```python
from build123d import *

# Parameters (mm, degrees)
F1_DEPTH = 60
F2_R     = 5
F3_R     = 25.0723290406
F4_DEPTH = 30


# Not quite as in the source:
# - a feature names something its author has since deleted; it is built from what else it names


with BuildPart() as f1:
    # F0 (on Front) → F1 (new body)
    with BuildSketch(Plane.XZ):
        with BuildLine():
            Line((21.3254676014, 72.3460770576), (-18.6745323986, 72.3460770576))
            ThreePointArc((-18.6745323986, 72.3460770576), (-39.8877358342, 63.5592804932), (-48.6745323986, 42.3460770576))
            Line((-48.6745323986, 42.3460770576), (-48.6745323986, 2.3460770576))
            ThreePointArc((-48.6745323986, 2.3460770576), (-39.8877358342, -18.867126378), (-18.6745323986, -27.6539229424))
            Line((-18.6745323986, -27.6539229424), (21.3254676014, -27.6539229424))
            ThreePointArc((21.3254676014, -27.6539229424), (42.538671037, -18.867126378), (51.3254676014, 2.3460770576))
            Line((51.3254676014, 2.3460770576), (51.3254676014, 42.3460770576))
            ThreePointArc((51.3254676014, 42.3460770576), (42.538671037, 63.5592804932), (21.3254676014, 72.3460770576))
        make_face()
    extrude(amount=F1_DEPTH)

    # F2
    f2_edges = [f1.edges().sort_by_distance(p)[0] for p in [
        (51.325468, -30, 42.346077),
        (21.325468, -30, 72.346077),
        (42.538671, 0, 63.55928),
        (42.538671, -60, 63.55928),
    ]]
    fillet(f2_edges, radius=F2_R)

    # F3 (on face) → F4 (cut)
    with BuildSketch(Plane.XZ.offset(60)):
        with Locations((-0.98494126, 18.3436237276)):
            Circle(F3_R)
    extrude(amount=-F4_DEPTH, mode=Mode.SUBTRACT)


solid = f1.part
```
Read the model definition and answer for the solid it produces. Units are mm, in the model's axes. A direction names the side the tool comes from. Give positions to 0.01 mm unless a question says otherwise; leave off trailing zeros. Loops run counter-clockwise (first coordinate to the right, second up) from the corner with the lowest first, then second, coordinate; pieces in that order, holes last.
Item 1: The part is cut by section C-C (y = -38.5). Write down the section's boundary in (x, z).
Item 2: Find the intervals of material crossed by line 1 along Z through (x, y) = (-9.5, -48.5); line 2 along Z through (x, y) = (-10, -43); line 3 along Y through (x, z) = (-11, 26.5), in increasing order.
Item 3: The mould has two halves that part along Z. Classify faces 3 (the cylindrical face through (22.93, -45.21, 25.87)), 4 (the cylindrical face through (49.9, -58.496, 22.626)), 5 (the cylindrical face through (1.045, -1.504, 70.92)): released by +Z, released by -Z, zero draft, split by the parting line, or undercut.
Item 4: Each of these flat-tipped pins is pushed along its axis until it touches: pin 1 Ø10 at (y, z) = (-29, -11.5) entering from +X; pin 2 Ø8 at (x, y) = (-32, -16) entering from +Z; pin 3 Ø12 at (y, z) = (-47, 54) entering from -X. Where does it stop, or does it pass through?
Item 5: The part is cut by section D-D (x = 17.5). Write down the section's boundary in (y, z).
Item 6: For faces 1 (the cylindrical face through (-47.249, -1.504, 22.066)), 2 (the flat face through (-1, -30, 19)), determine the directions among +Z, -Z, +X, -X, +Y, -Y from which every point of the face is accessible in a straight line to the end or side of a thin tool.
Item 7: The part is cut by section A-A (y = -27.5). Write down the section's boundary in (x, z).
Item 8: The part is cut by section B-B (z = 6.5). Write down the section's boundary in (x, y), and give its area (3 significant figures).
Taken from the geometry:
1. outline: (-48.67, 2.35) arc R30 ccw to (-18.67, -27.65) - (21.33, -27.65) arc R30 ccw to (51.33, 2.35) - (51.33, 42.35) arc R30 ccw to (21.33, 72.35) - (-18.67, 72.35) arc R30 ccw to (-48.67, 42.35) - close; hole circle Ø50.14 at (-0.98, 18.34)
2. line 1: z = -27.65 to -5.24, 41.93 to 72.35
2. line 2: z = -27.65 to -5.05, 41.74 to 72.35
2. line 3: y = -30 to 0
3. face 3: undercut
3. face 4: zero draft
3. face 5: released by +Z
4. pin 1: stops at x = 49.99
4. pin 2: stops at z = 70.86
4. pin 3: stops at x = -48.14
5. outline: (-60, -22.65) arc R5 ccw to (-55, -27.65) - (-5, -27.65) arc R5 ccw to (0, -22.65) - (0, 67.35) arc R5 ccw to (-5, 72.35) - (-55, 72.35) arc R5 ccw to (-60, 67.35) - (-60, 35.28) - (-30, 35.28) - (-30, 1.4) - (-60, 1.4) - close
6. face 1: +Z, -Z, -X, +Y
6. face 2: -Y
7. outline: (-48.67, 2.35) arc R30 ccw to (-18.67, -27.65) - (21.33, -27.65) arc R30 ccw to (51.33, 2.35) - (51.33, 42.35) arc R30 ccw to (21.33, 72.35) - (-18.67, 72.35) arc R30 ccw to (-48.67, 42.35) - close
8. outline: (-48.67, -55) arc R5 ccw to (-43.67, -60) - (-23.08, -60) - (-23.08, -30) - (21.11, -30) - (21.11, -60) - (46.33, -60) arc R5 ccw to (51.33, -55) - (51.33, -5) arc R5 ccw to (46.33, 0) - (-43.67, 0) arc R5 ccw to (-48.67, -5) - close
8. area: 4,650 mm2
